from build123d import *

# Parameters (mm, degrees)
F1_W           = 25.4
F1_H           = 25.4
F3_DEPTH       = 46.228
F4_DEPTH       = 23.876
F6_D           = 11
F6_DEPTH       = 12.7
F6_CSINK_D     = 22.4
F6_CSINK_ANGLE = 90
F6_TIP         = 3.3047334047
F8_D           = 5.5
F8_DEPTH       = 12.7
F8_CSINK_D     = 11.2
F8_CSINK_ANGLE = 90
F8_TIP         = 1.6523667023


with BuildPart() as f3:
    # F1 (on face) → F3 (new body, symmetric)
    with BuildSketch(Plane.XZ):
        with Locations((-12.7, 25.4)):
            Rectangle(F1_W, F1_H)
    extrude(amount=F3_DEPTH, both=True)

    # F2 (on face) → F4 (join, symmetric)
    with BuildSketch(Plane.XZ):
        Polygon((0, 12.7), (-25.4, 12.7), (-25.4, -12.7), (25.4, -12.7), (25.4, 12.7), align=None)
    extrude(amount=F4_DEPTH, both=True)

    # F6
    with Locations(Plane(origin=(0, 0, -12.7), x_dir=(1, 0, 0), z_dir=(0, 0, -1))):
        with Locations((0, -1.524)):
            CounterSinkHole(F6_D / 2, F6_CSINK_D / 2, depth=F6_DEPTH, counter_sink_angle=F6_CSINK_ANGLE)
            with Locations((0, 0, -(F6_DEPTH + F6_TIP / 2))):  # 118° drill point
                Cone(0, F6_D / 2, F6_TIP, mode=Mode.SUBTRACT)

    # F8
    with Locations(Plane.XY.offset(12.7)):
        with Locations((17.78, -16.256)):
            CounterSinkHole(F8_D / 2, F8_CSINK_D / 2, depth=F8_DEPTH, counter_sink_angle=F8_CSINK_ANGLE)
            with Locations((0, 0, -(F8_DEPTH + F8_TIP / 2))):  # 118° drill point
                Cone(0, F8_D / 2, F8_TIP, mode=Mode.SUBTRACT)


solid = f3.part
Work out the finished part from the listing and answer in its coordinate system (mm). A direction names the side the tool comes from. Give positions to 0.01 mm unless a question says otherwise; leave off trailing zeros. Loops run counter-clockwise (first coordinate to the right, second up) from the corner with the lowest first, then second, coordinate; pieces in that order, holes last. Notation, with made-up numbers: (-22, -27.75) - (-9, -27.75) arc R26 ccw to (-9, 1.25) - close; hole circle Ø9 at (29, -37.75). An arc over 180 degrees is marked (long way). Answer in a Markdown table with one row per item. Add a question column.
Q1. Determine the mould class of faces 5 (the flat face through (-25.4, -1, 19)), 6 (the flat face through (0, -11, -12.7)), 7 (the conical face through (-0.21, 2.46, 2.73)) for opening direction X: released by +X, released by -X, zero draft, split by the parting line, or undercut.
Q2. Each of these flat-tipped pins is pushed along its axis until it touches: P1, Ø4, axis at x = -6, y = -29, coming from the -Z side; P2, Ø20.5, axis at x = 12.5, z = 5, coming from the -Y side; P3, Ø12.5, axis at x = -10, z = -3.5, coming from the +Y side. Where does it stop, or does it pass through?
Q3. Consider line 1 along Y through (x, z) = (17.78, 3.75); line 2 along Y through (x, z) = (0, -4.75); line 3 along Z through (x, y) = (15, 1). Determine where each line is inside the solid, lowest interval first.
Q4. The part is cut by section A-A (z = -4). Determine the outline of the cut face in (x, y).
Q5. The part is cut by section C-C (z = 20.5). Determine the outline of the cut face in (x, y), and give its area (3 significant figures).
Q6. The part is cut by section B-B (x = -22). Determine the outline of the cut face in (y, z).
Q7. A tool of negligible diameter and unlimited length cuts with its end or side. For faces 1 (the flat face through (0, -23.876, 0)), 2 (the cylindrical face through (5.495, 1.282, -3.451)), 3 (the flat face through (-13, 35, 12.7)), 4 (the flat face through (13, 0, 12.7)), from which of +Z, -Z, +X, -X, +Y, -Y can it reach the whole face along a straight path? Write none if from no direction.
Q8. The part is cut by section D-D (z = 6.5). Determine the outline of the cut face in (x, y).
Solution:
| question | item | result |
|---|---|---|
| 1 | face 5 | released by -X |
| 1 | face 6 | zero draft |
| 1 | face 7 | undercut |
| 2 | P1 | stops at z = 12.7 |
| 2 | P2 | stops at y = -23.88 |
| 2 | P3 | stops at y = 23.88 |
| 3 | line 1 | y = -23.88 to -19.01, -13.51 to 23.88 |
| 3 | line 2 | y = -23.88 to -3.98, 7.02 to 23.88 |
| 3 | line 3 | z = -12.7 to 12.7 |
| 4 | outline | (-25.4, -23.88) - (25.4, -23.88) - (25.4, 23.88) - (-25.4, 23.88) - close; hole circle Ø11 at (0, 1.52) |
| 5 | outline | (-25.4, -46.23) - (0, -46.23) - (0, 46.23) - (-25.4, 46.23) - close |
| 5 | area | 2,350 mm² |
| 6 | outline | (-46.23, 12.7) - (-23.88, 12.7) - (-23.88, -12.7) - (23.88, -12.7) - (23.88, 12.7) - (46.23, 12.7) - (46.23, 38.1) - (-46.23, 38.1) - close |
| 7 | face 1 | -Z, +X, -X, -Y |
| 7 | face 2 | -Z |
| 7 | face 3 | -Z, +X, -X, +Y |
| 7 | face 4 | +Z, +X, +Y, -Y |
| 8 | outline | (-25.4, -23.88) - (25.4, -23.88) - (25.4, 23.88) - (-25.4, 23.88) - close; hole circle Ø5.5 at (17.78, -16.26) |
